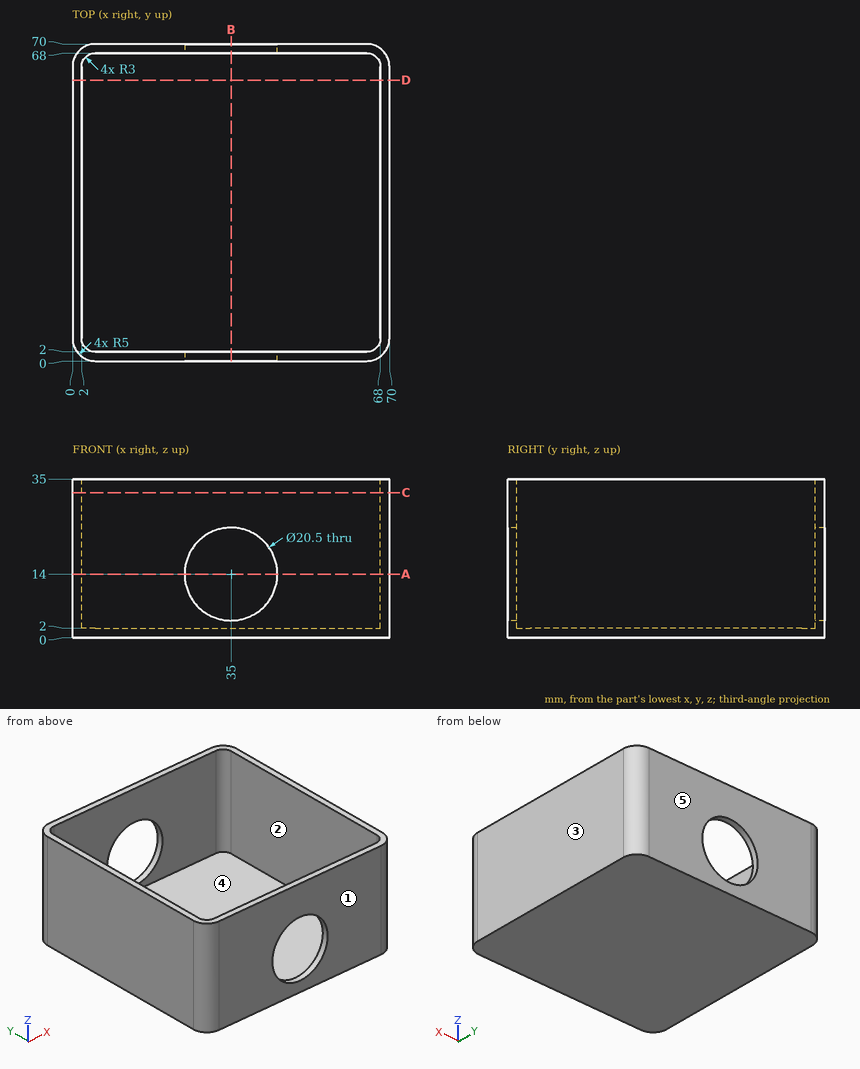
Study the drawing (mm; zero at the part's minimum x, y, z) and answer. A direction names the side the tool comes from. Give positions to 0.01 mm unless a question says otherwise; leave off trailing zeros. Loops run counter-clockwise (first coordinate to the right, second up) from the corner with the lowest first, then second, coordinate; pieces in that order, holes last. Notation, with made-up numbers: (55.25, 5) - (90.25, 5) arc R19 cw to (90.25, 25) - close; hole circle Ø8 at (2, 30.25). An arc over 180 degrees is marked (long way). One line per question, with ' | ' between items.
(1) A tool of negligible diameter and unlimited length cuts with its end or side. For the marked faces 4 and 5, from which of +Z, -Z, +X, -X, +Y, -Y can it reach the whole face along a straight path? Write none if from no direction.
Recorded:
face 4: +Z | face 5: +Z, -Z, +X, -X, +Y
(2) Straight lines are drawn through the part: probe 1 along Y at (x, z) = (64.5, 7); probe 2 along Z at (x, y) = (35, 0.85). For each, find the intervals that lie inside material, in ascending order.
Recorded:
probe 1: y = 0 to 2, 68 to 70 | probe 2: z = 0 to 3.75, 24.25 to 35
(3) The part is cut by section D-D (y = 62). Write down the section's boundary in (x, z), then the cut area to 3 significant figures.
Recorded:
outline: (0, 0) - (70, 0) - (70, 35) - (68, 35) - (68, 2) - (2, 2) - (2, 35) - (0, 35) - close | area: 272 mm²
(4) The part is cut by section C-C (z = 32). Write down the section's boundary in (x, y), then the cut area to 3 significant figures.
Recorded:
outline: (0, 5) arc R5 ccw to (5, 0) - (65, 0) arc R5 ccw to (70, 5) - (70, 65) arc R5 ccw to (65, 70) - (5, 70) arc R5 ccw to (0, 65) - close; hole (2, 5) arc R3 ccw to (5, 2) - (65, 2) arc R3 ccw to (68, 5) - (68, 65) arc R3 ccw to (65, 68) - (5, 68) arc R3 ccw to (2, 65) - close | area: 530 mm²
(5) The mould has two halves that part along X. Classify the marked faces 1, 2 and 3: +X half, -X half, draft (parallel to the pull), parting line (faces both ways), or undercut.
Recorded:
face 1: draft | face 2: undercut | face 3: +X half
(6) The part is cut by section A-A (z = 14). Write down the section's boundary in (x, y), then the cut area to 3 significant figures.
Recorded:
outline: (0, 5) arc R5 ccw to (5, 0) - (24.75, 0) - (24.75, 2) - (5, 2) arc R3 cw to (2, 5) - (2, 65) arc R3 cw to (5, 68) - (24.75, 68) - (24.75, 70) - (5, 70) arc R5 ccw to (0, 65) - close; (45.25, 0) - (65, 0) arc R5 ccw to (70, 5) - (70, 65) arc R5 ccw to (65, 70) - (45.25, 70) - (45.25, 68) - (65, 68) arc R3 cw to (68, 65) - (68, 5) arc R3 cw to (65, 2) - (45.25, 2) - close | area: 448 mm²
(7) The part is cut by section B-B (x = 35). Write down the section's boundary in (y, z), then the cut area to 3 significant figures.
Recorded:
outline: (0, 0) - (70, 0) - (70, 3.75) - (68, 3.75) - (68, 2) - (2, 2) - (2, 3.75) - (0, 3.75) - close; (0, 24.25) - (2, 24.25) - (2, 35) - (0, 35) - close; (68, 24.25) - (70, 24.25) - (70, 35) - (68, 35) - close | area: 190 mm²
(8) Each of these flat-tipped pins is pushed along its axis until it touches: pin 1 Ø4 at (x, y) = (12, 53) entering from -Z; pin 2 Ø12 at (x, y) = (18, 51) entering from +Z. Where does it stop, or does it pass through?
Recorded:
pin 1: stops at z = 0 | pin 2: stops at z = 2
